Here's how the part is built. I have some questions about the finished solid (model axes, mm). Give positions to 0.01 mm unless a question says otherwise; leave off trailing zeros. Write each loop counter-clockwise with the first axis right and the second up, starting at its lowest first coordinate (ties: lowest second). Pieces come first, ordered by that corner, then holes. Notation, with made-up numbers: (-0.5, 82) -> (35.5, 82) arc R22 cw to (35.5, 106) -> close; hole circle Ø9 at (-7, 76.25). An arc over 180 degrees is marked (long way). Return JSON: item names as keys, results as strings.
from build123d import *

# Parameters (mm, degrees)
BOSS_EXTRUDE1_DEPTH = 6
BOSS_EXTRUDE2_DEPTH = 3


with BuildPart() as part:
    # Sketch1 → Boss-Extrude1 (new body)
    with BuildSketch(Plane(origin=(0, 0, 0), x_dir=(1, 0, 0), z_dir=(0, 1, 0))):
        Polygon((0, 35), (-35, 35), (0, 0), align=None)
    extrude(amount=BOSS_EXTRUDE1_DEPTH)

    # Sketch1_3 → Boss-Extrude2 (add)
    with BuildSketch(Plane(origin=(0, 0, 0), x_dir=(1, 0, 0), z_dir=(0, 1, 0))):
        Polygon((0, 35), (0, 27), (4, 31), (4, 39), (-4, 39), (-8, 35), align=None)
    extrude(amount=BOSS_EXTRUDE2_DEPTH)


solid = part.part
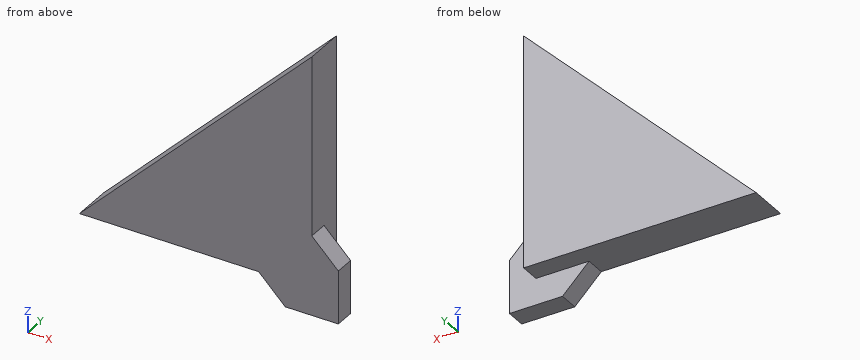
1. Suppose I cut it at D-D, the plane z = -12. List the corners of the cut face in (x, y) for me.
Taken from the geometry:
{"outline": "(-12, 0) -> (0, 0) -> (0, 6) -> (-12, 6) -> close"}
2. If I drill on line 1 (Z direction, x = -31, y = 4.75); line 2 (Z direction, x = -8, y = 1.4); line 3 (X direction, y = 3.85, z = -33), over which ranges is the centre line in solid material (lowest first)? Write a range as [from, to].
Taken from the geometry:
{"line 1": "z = [-35, -31]", "line 2": "z = [-35, -8]", "line 3": "x = [-33, 0]"}
3. Suppose I cut it at B-B, the plane z = -33.5. List the corners of the cut face in (x, y) for me.
Taken from the geometry:
{"outline": "(-33.5, 0) -> (4, 0) -> (4, 3) -> (0, 3) -> (0, 6) -> (-33.5, 6) -> close"}
4. Suppose I cut it at C-C, the plane x = -1.5. List the corners of the cut face in (y, z) for me, and give its area (3 significant figures).
Taken from the geometry:
{"outline": "(0, -39) -> (3, -39) -> (3, -35) -> (6, -35) -> (6, -1.5) -> (0, -1.5) -> close", "area": "213 mm²"}
5. For pin 1 Ø2 at (x, y) = (-23, 3.5) entering from +Z; pin 2 Ø3 at (y, z) = (3, -17.5) entering from +X; pin 3 Ø1.5 at (y, z) = (2, -25) entering from -X, each with a flat end and sliding along its axis, tell me the tip position at first contact or that it passes through.
Taken from the geometry:
{"pin 1": "stops at z = -22", "pin 2": "stops at x = 0", "pin 3": "stops at x = -25.75"}
6. Suppose I cut it at A-A, the plane y = 1.35. List the corners of the cut face in (x, z) for me, and give its area (4 significant figures).
Taken from the geometry:
{"outline": "(-35, -35) -> (-8, -35) -> (-4, -39) -> (4, -39) -> (4, -31) -> (0, -27) -> (0, 0) -> close", "area": "676.5 mm²"}
